Verification items for the finished model (mm, model axes). Face numbers are marked on the shaded views. A direction names the side the tool comes from. Coordinates: 2 decimals unless noted, no trailing zeros. Order: outer loops, then holes, each group sorted by start corner. A loop starts at its lowest first (then second) coordinate and runs counter-clockwise, first axis right, second up. Notation, with made-up numbers: (-33.5, 56.25) -> (-26.5, 56.25) arc R23 ccw to (-26.5, 90.25) -> close; hole circle Ø4 at (61.5, 8.25). An arc over 180 degrees is marked (long way). Write item = value, one per line. Start each with the question number.
from build123d import *

# Parameters (mm, degrees)
CUT_EXTRUDE2_START = -5
CUT_EXTRUDE2_DEPTH = 5
CIRPATTERN1_COUNT  = 11


with BuildPart() as part:
    # Sketch4 → Revolve1 (revolve)
    with BuildSketch(Plane(origin=(0, 0, 0), x_dir=(0, 0, -1), z_dir=(1, 0, 0))):
        with BuildLine():
            Line((0, 0), (0, 26.1))
            Line((0, 26.1), (1, 26.1))
            Line((1, 26.1), (1, 26))
            Line((1, 26), (2, 26))
            Line((2, 26), (2, 22))
            Line((2, 22), (1, 22))
            Line((1, 22), (1, 20))
            Line((1, 20), (3.5, 20))
            ThreePointArc((3.5, 20), (3.853553391, 19.853553391), (4, 19.5))
            Line((4, 19.5), (4, 0))
            Line((4, 0), (0, 0))
        make_face()
    revolve(axis=Axis((0, 0, 0), (0, 1, 0)))

    # Sketch5 → Cut-Extrude2 (cut)
    with BuildSketch(Plane(origin=(0, 26, 0), x_dir=(1, 0, 0), z_dir=(0, 1, 0)).offset(CUT_EXTRUDE2_START)):
        with BuildLine():
            ThreePointArc((0.332507409, 1.972166023), (0.190245846, 1.670802314), (0.1, 1.35))
            ThreePointArc((0.1, 1.35), (0, 1.25), (-0.1, 1.35))
            ThreePointArc((-0.1, 1.35), (-0.190245846, 1.670802314), (-0.332507409, 1.972166023))
            ThreePointArc((-0.332507409, 1.972166023), (0, 2), (0.332507409, 1.972166023))
        make_face()
    cut_extrude2 = extrude(amount=CUT_EXTRUDE2_DEPTH, mode=Mode.SUBTRACT)

    # CirPattern1: Cut-Extrude2 ×11 about axis
    cirpattern1_axis = Axis((0, 0, 0), (0, 1, 0))
    for i in range(1, CIRPATTERN1_COUNT):
        add(cut_extrude2.rotate(cirpattern1_axis, i * 360 / CIRPATTERN1_COUNT), mode=Mode.SUBTRACT)


solid = part.part
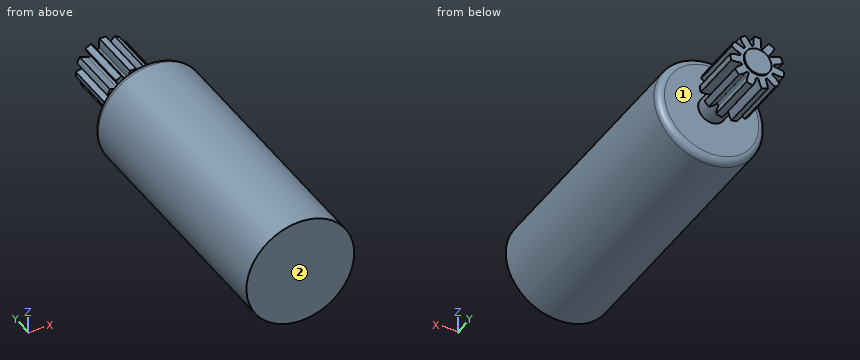
Item 1: Tool access check on the marked faces 1 and 2. Record the directions out of +Z, -Z, +X, -X, +Y, -Y that give a thin tool (end or side, any length) a straight path to the whole face; none if there is none.
Item 2: Section check A-A (y = 7.5). Record the boundary of the cut face in (x, z), then the cut area to 3 significant figures.
Item 3: Thickness scan on line 1 (Y direction, x = 3, z = 1); line 2 (Z direction, x = 3.5, y = 14.75); line 3 (X direction, y = 6, z = 0.25). Record the ranges inside material, lowest first.
Item 4: Gauge pin test, flat ends, axial feed: P1, Ø3, axis at x = -2, z = -0.5, coming from the +Y side; P2, Ø3, axis at y = 10.5, z = 2, coming from the -X side; P3, Ø1, axis at y = 17, z = -2, coming from the -X side. Record the tip position at first contact, or that the pin passes through.
Filled sheet:
q1.face_1 = none
q1.face_2 = +Z, -Z, +X, -X, -Y
q2.outline = circle Ø8 at (0, 0)
q2.area = 50.3 mm^2
q3.line_1 = 0 to 20
q3.line_2 = -1.94 to 1.94
q3.line_3 = -3.99 to 3.99
q4.P1 = 26.1
q4.P2 = -3.97
q4.P3 = -3.71
